Geometry check sheet. Reference: the model listing, model coordinates, mm. A direction names the side the tool comes from. Round coordinates to 2 decimals unless told otherwise and drop trailing zeros. Write each loop counter-clockwise with the first axis right and the second up, starting at its lowest first coordinate (ties: lowest second). Pieces come first, ordered by that corner, then holes.
from build123d import *

# Parameters (mm, degrees)
F0_R      = 20
F1_DEPTH  = 60
F0_R_2    = 5
F2_DEPTH  = 15
F3_DEPTH  = 60
F4_DEPTH  = 45
F5_DEPTH  = 15
F7_DEPTH  = 30
F9_DEPTH  = 5
F10_R     = 7.5
F11_DEPTH = 15


with BuildPart() as f1:
    # F0 (on Top) → F1 (new body)
    with BuildSketch(Plane.XY):
        with BuildLine():
            ThreePointArc((25, -16.5831239518), (28.7228132327, -8.6602540378), (30, 0))
            ThreePointArc((30, 0), (22.9128784748, 19.364916731), (5, 29.5803989155))
            ThreePointArc((5, 29.5803989155), (0, 30), (-5, 29.5803989155))
            ThreePointArc((-5, 29.5803989155), (-22.9128784748, 19.364916731), (-30, 0))
            ThreePointArc((-30, 0), (-28.7228132327, -8.6602540378), (-25, -16.5831239518))
            ThreePointArc((-25, -16.5831239518), (-16.3472410247, -25.1548744954), (-5, -29.5803989155))
            ThreePointArc((-5, -29.5803989155), (0, -30), (5, -29.5803989155))
            ThreePointArc((5, -29.5803989155), (16.3472410247, -25.1548744954), (25, -16.5831239518))
        make_face()
        Circle(F0_R, mode=Mode.SUBTRACT)
    extrude(amount=F1_DEPTH)

    # F0 (on Top) → F2 (join)
    with BuildSketch(Plane.XY):
        with BuildLine():
            Line((25, -75), (25, -16.5831239518))
            ThreePointArc((25, -16.5831239518), (16.3472410247, -25.1548744954), (5, -29.5803989155))
            Line((5, -29.5803989155), (5, -54.5803989155))
            Line((5, -54.5803989155), (0, -54.5803989155))
            Line((0, -54.5803989155), (-5, -54.5803989155))
            Line((-5, -54.5803989155), (-5, -29.5803989155))
            ThreePointArc((-5, -29.5803989155), (-16.3472410247, -25.1548744954), (-25, -16.5831239518))
            Line((-25, -16.5831239518), (-25, -75))
            ThreePointArc((-25, -75), (0, -100), (25, -75))
        make_face()
        with Locations((0, -75)):
            Circle(F0_R_2, mode=Mode.SUBTRACT)
        with BuildLine():
            Line((5, -54.5803989155), (5, -29.5803989155))
            ThreePointArc((5, -29.5803989155), (0, -30), (-5, -29.5803989155))
            Line((-5, -29.5803989155), (-5, -54.5803989155))
            Line((-5, -54.5803989155), (0, -54.5803989155))
            Line((0, -54.5803989155), (5, -54.5803989155))
        make_face()
    extrude(amount=F2_DEPTH)

    # F0 (on Top) → F3 (join)
    with BuildSketch(Plane.XY):
        with BuildLine():
            ThreePointArc((-30, 0), (-22.9128784748, 19.364916731), (-5, 29.5803989155))
            Line((-5, 29.5803989155), (-5, 60))
            Line((-5, 60), (-30, 60))
            Line((-30, 60), (-30, 0))
        make_face()
        with BuildLine():
            ThreePointArc((-5, 29.5803989155), (0, 30), (5, 29.5803989155))
            Line((5, 29.5803989155), (5, 60))
            Line((5, 60), (30, 60))
            Line((30, 60), (30, 75))
            Line((30, 75), (-30, 75))
            Line((-30, 75), (-30, 60))
            Line((-30, 60), (-5, 60))
            Line((-5, 60), (-5, 29.5803989155))
        make_face()
        with BuildLine():
            ThreePointArc((5, 29.5803989155), (22.9128784748, 19.364916731), (30, 0))
            Line((30, 0), (30, 60))
            Line((30, 60), (5, 60))
            Line((5, 60), (5, 29.5803989155))
        make_face()
    extrude(amount=F3_DEPTH)

    # F0 (on Top) → F4 (join)
    with BuildSketch(Plane.XY):
        with BuildLine():
            ThreePointArc((25, -16.5831239518), (28.7228132327, -8.6602540378), (30, 0))
            ThreePointArc((30, 0), (22.9128784748, 19.364916731), (5, 29.5803989155))
            ThreePointArc((5, 29.5803989155), (0, 30), (-5, 29.5803989155))
            ThreePointArc((-5, 29.5803989155), (-22.9128784748, 19.364916731), (-30, 0))
            ThreePointArc((-30, 0), (-28.7228132327, -8.6602540378), (-25, -16.5831239518))
            ThreePointArc((-25, -16.5831239518), (-16.3472410247, -25.1548744954), (-5, -29.5803989155))
            ThreePointArc((-5, -29.5803989155), (0, -30), (5, -29.5803989155))
            ThreePointArc((5, -29.5803989155), (16.3472410247, -25.1548744954), (25, -16.5831239518))
        make_face()
        Circle(F0_R, mode=Mode.SUBTRACT)
        with BuildLine():
            ThreePointArc((-5, 29.5803989155), (0, 30), (5, 29.5803989155))
            Line((5, 29.5803989155), (5, 60))
            Line((5, 60), (30, 60))
            Line((30, 60), (30, 75))
            Line((30, 75), (-30, 75))
            Line((-30, 75), (-30, 60))
            Line((-30, 60), (-5, 60))
            Line((-5, 60), (-5, 29.5803989155))
        make_face()
    extrude(amount=F4_DEPTH)

    # F0 (on Top) → F5 (cut)
    with BuildSketch(Plane.XY):
        with BuildLine():
            ThreePointArc((-30, 0), (-22.9128784748, 19.364916731), (-5, 29.5803989155))
            Line((-5, 29.5803989155), (-5, 60))
            Line((-5, 60), (-30, 60))
            Line((-30, 60), (-30, 0))
        make_face()
        with BuildLine():
            ThreePointArc((-5, 29.5803989155), (0, 30), (5, 29.5803989155))
            Line((5, 29.5803989155), (5, 60))
            Line((5, 60), (30, 60))
            Line((30, 60), (30, 75))
            Line((30, 75), (-30, 75))
            Line((-30, 75), (-30, 60))
            Line((-30, 60), (-5, 60))
            Line((-5, 60), (-5, 29.5803989155))
        make_face()
        with BuildLine():
            ThreePointArc((5, 29.5803989155), (22.9128784748, 19.364916731), (30, 0))
            Line((30, 0), (30, 60))
            Line((30, 60), (5, 60))
            Line((5, 60), (5, 29.5803989155))
        make_face()
    extrude(amount=F5_DEPTH, mode=Mode.SUBTRACT)

    # F6 (on face) → F7 (cut)
    with BuildSketch(Plane.XY.offset(60)):
        with BuildLine():
            Line((-5, 29.5803989155), (-5, 60))
            Line((-5, 60), (-30, 60))
            Line((-30, 60), (-30, 0))
            ThreePointArc((-30, 0), (-22.9128784748, 19.364916731), (-5, 29.5803989155))
        make_face()
        with BuildLine():
            Line((5, 60), (5, 29.5803989155))
            ThreePointArc((5, 29.5803989155), (22.9128784748, 19.364916731), (30, 0))
            Line((30, 0), (30, 60))
            Line((30, 60), (5, 60))
        make_face()
    extrude(amount=-F7_DEPTH, mode=Mode.SUBTRACT)

    # F8 (on Right) → F9 (join, symmetric)
    with BuildSketch(Plane.YZ):
        Polygon((-55.0730913877, 15), (-30.0730913877, 15), (-30.0730913877, 60), align=None)
    extrude(amount=F9_DEPTH, both=True)

    # F10 (on face) → F11 (cut)
    with BuildSketch(Plane.XZ.offset(-60)):
        with Locations((-17.7129209042, 45)):
            Circle(F10_R)
        with Locations((17.2870790958, 45)):
            Circle(F10_R)
    extrude(amount=-F11_DEPTH, mode=Mode.SUBTRACT)


solid = f1.part
1. Scan lines: line 1 along Y through (x, z) = (-3, 22); line 2 along X through (y, z) = (-37, 35); line 3 along Y through (x, z) = (-25, 43). Record each from-to range of solid material in increasing order.
2. Section check C-C (x = 0). Record the cut outline in (y, z), plus the area to 3 significant figures.
3. Section check B-B (y = -78). Record the cut outline in (x, z), plus the area to 3 significant figures.
4. Section check A-A (z = 33.5). Record the cut outline in (x, y), plus the area to 3 significant figures.
5. Section check D-D (z = 45). Record the cut outline in (x, y).
6. Depth check by flat-ended pin: pin 1 Ø19.5 at (x, z) = (17.29, 45) entering from -Y; pin 2 Ø1.5 at (x, y) = (23, -62.5) entering from +Z; pin 3 Ø5 at (x, y) = (6.5, -36) entering from +Z. Enter the tip coordinate at first touch or a pass-through.
7. Access from +Z, -Z, +X, -X, +Y, -Y to the whole of each face (thin tool, end or side, straight path). Record for faces 5 (the face through (25, -46, 7)), 6 (the face through (26, 60, 45)), 7 (the face through (-5, 45, 45)), 8 (the face through (-5, -37, 28)).
8. Release check for a two-part mould opening along X. For faces 1 (the face through (-1.08, -79.88, 7.4)), 2 (the face through (5, -37, 28)), 3 (the face through (-25, -45, 7)), 4 (the face through (15.66, 67.4, 37.68)) record: +X half, -X half, draft (parallel to the pull), parting line (faces both ways), or undercut.
Results below:
1. line 1: y = -51.18 to -30.07, -29.85 to -19.77, 19.77 to 75
1. line 2: x = -5 to 5
1. line 3: y = -16.58 to 16.58, 60 to 75
2. outline: (-100, 0) - (-80, 0) - (-80, 15) - (-100, 15) - close; (-70, 0) - (-20, 0) - (-20, 60) - (-30, 60) - (-30, 15) - (-30.07, 15) - (-30.07, 60) - (-55.07, 15) - (-70, 15) - close; (20, 0) - (30, 0) - (30, 15) - (75, 15) - (75, 60) - (20, 60) - close
2. area: 4,690 mm2
3. outline: (-24.82, 0) - (-4, 0) - (-4, 15) - (-24.82, 15) - close; (4, 0) - (24.82, 0) - (24.82, 15) - (4, 15) - close
3. area: 625 mm2
4. outline: (-30, 60) - (-5, 60) - (-5, 29.58) arc R30 ccw (long way) to (5, 29.58) - (5, 60) - (30, 60) - (30, 75) - (-30, 75) - close; (-5, -44.8) - (5, -44.8) - (5, -30.07) - (-5, -30.07) - close; hole circle Ø40 at (0, 0)
4. area: 2,920 mm2
5. outline: (-30, 60) - (-25.21, 60) - (-25.21, 75) - (-30, 75) - close; (-10.21, 60) - (-5, 60) - (-5, 29.58) arc R30 ccw (long way) to (5, 29.58) - (5, 60) - (9.79, 60) - (9.79, 75) - (-10.21, 75) - close; (-5, -38.41) - (5, -38.41) - (5, -30.07) - (-5, -30.07) - close; (24.79, 60) - (30, 60) - (30, 75) - (24.79, 75) - close; hole circle Ø40 at (0, 0)
6. pin 1: stops at y = -29.04
6. pin 2: stops at z = 15
6. pin 3: stops at z = 52.93
7. face 5: +Z, -Z, +X, -Y
7. face 6: +Z, +X
7. face 7: +Z, -X
7. face 8: +Z, -X, -Y
8. face 1: undercut
8. face 2: +X half
8. face 3: -X half
8. face 4: undercut
